Design review of the part built by this model. Coordinates are the model's own, in mm. A direction names the side the tool comes from. Coordinates: 2 decimals unless noted, no trailing zeros. Loops run counter-clockwise (first coordinate to the right, second up) from the corner with the lowest first, then second, coordinate; pieces in that order, holes last. Notation, with made-up numbers: M 83,66.5 L 124,66.5 A25 ccw 124,85.5 Z; hole C -6.75,12 d1. An arc over 180 degrees is marked long. Put each result on its own line as item: value. Start each with the question number.
(1) Take a section at C-C, the plane x = -53.5. Give the boundary of the cut face in (y, z).
(2) For faces 4 (the cylindrical face through (-48.91, -21.07, 7.19)), 5 (the flat face through (52, -28, 23.5)), 6 (the flat face through (-1, -33.4, 22)), list the 3-axis set-ups (+Z, -Z, +X, -X, +Y, -Y) from which the entire face can be reached by the end or side of a thin tool; tool diameter is ignored.
(3) For probe 1 along X at (y, z) = (-22, 6); probe 2 along X at (y, z) = (0, 2.05); probe 3 along Y at (x, z) = (51.5, 22), list the stretches that pass through material, from the lowest coordinate up. Write a range as [from, to].
(4) The part is to be moulded in two halves that separate along X. For faces 1 (the cylindrical face through (-43.624, 22.024, 7.19)), 2 (the cylindrical face through (57.321, 0.22, 27.745)), 3 (the flat face through (-49.34, 23.03, 11.5)), say which applies: +X half, -X half, draft (parallel to the pull), parting line (faces both ways), or undercut.
(5) Clearance check with flat-ended pins moving along their axes: pin 1 (2.5 mm diameter, centred on x = -49.5, y = -22.5, fed in from +Z); pin 2 (6 mm diameter, centred on x = 20, y = 20, fed in from +Z); pin 3 (3 mm diameter, centred on x = 53.5, y = 28.1, fed in from +Z); pin 4 (2 mm diameter, centred on x = -48.8, y = 0, fed in from -Z). State where each tip first meets the part, or that it passes through.
(6) Take a section at A-A, the plane z = 9. Count the separate pieces of the cut face and the enclosed holes in it, then the cut area to 3 significant figures.
(7) Take a section at D-D, the plane y = 28.1. Give the boundary of the cut face in (x, z).
(8) Take a section at B-B, the plane z = 36.5. Give the boundary of the cut face in (x, y).
```python
from build123d import *

# Parameters (mm, degrees)
SCHIZZO1_W                           = 117.6
SCHIZZO1_H                           = 66.8
ESTRUSIONE_ESTRUSIONE1_DEPTH         = 3
SCHIZZO2_W                           = 117.6
SCHIZZO2_H                           = 66.8
SCHIZZO2_W_2                         = 111.6
SCHIZZO2_H_2                         = 60.8
ESTRUSIONE_FORI_COVER_DEPTH          = 40.5
SCHIZZO4_R                           = 4
SCHIZZO4_R_2                         = 1.75
ESTRUSIONE_FORI_PCB_DEPTH            = 8.5
SCHIZZO7_R                           = 3.5
ESTRUSIONE_FORI_CHASSIS_DEPTH        = 1
SCHIZZO8_R                           = 1.85
TAGLIO_ESTRUSIONE2_DEPTH             = 79.82417142
TAGLIO_ESTRUSIONE2_DIRECTION_2_REACH = 80.824
RACCORDO3_R                          = 2
RACCORDO4_R                          = 2
RACCORDO5_R                          = 2
RACCORDO6_R                          = 2
RACCORDO7_R                          = 2
SCHIZZO9_R                           = 1.2
ESTRUSIONE_ESTRUSIONE6_DEPTH         = 20
TAGLIO_FORO_CAVI_REACH               = 131.76
SCHIZZO11_R                          = 5


with BuildPart() as part:
    # Schizzo1 → Estrusione-Estrusione1 (new body)
    with BuildSketch(Plane.XY):
        Rectangle(SCHIZZO1_W, SCHIZZO1_H)
    extrude(amount=ESTRUSIONE_ESTRUSIONE1_DEPTH)

    # Schizzo2 → Estrusione- Fori Cover (add)
    with BuildSketch(Plane.XY.offset(3)):
        Rectangle(SCHIZZO2_W, SCHIZZO2_H)
        Rectangle(SCHIZZO2_W_2, SCHIZZO2_H_2, mode=Mode.SUBTRACT)
    extrude(amount=ESTRUSIONE_FORI_COVER_DEPTH)

    # Schizzo4 → Estrusione- Fori PCB (add)
    # profile 1 of 4: a face of its own
    with BuildSketch(Plane.XY.offset(3)):
        with Locations(Location((-47.62, 22.2, 0), (0, 0, 180))):
            Circle(SCHIZZO4_R)
        with Locations((-47.62, 22.2)):
            Circle(SCHIZZO4_R_2, mode=Mode.SUBTRACT)
    # profile 2 of 4: a face of its own
    with BuildSketch(Plane.XY.offset(3)):
        with Locations(Location((47.63, 22.2, 0), (0, 0, 180))):
            Circle(SCHIZZO4_R)
        with Locations((47.63, 22.2)):
            Circle(SCHIZZO4_R_2, mode=Mode.SUBTRACT)
    # profile 3 of 4: a face of its own
    with BuildSketch(Plane.XY.offset(3)):
        with Locations(Location((47.63, -22.25, 0), (0, 0, 180))):
            Circle(SCHIZZO4_R)
        with Locations((47.63, -22.25)):
            Circle(SCHIZZO4_R_2, mode=Mode.SUBTRACT)
    # profile 4 of 4: a face of its own
    with BuildSketch(Plane.XY.offset(3)):
        with Locations(Location((-47.62, -22.25, 0), (0, 0, 180))):
            Circle(SCHIZZO4_R)
        with Locations((-47.62, -22.25)):
            Circle(SCHIZZO4_R_2, mode=Mode.SUBTRACT)
    extrude(amount=ESTRUSIONE_FORI_PCB_DEPTH)

    # Schizzo7 → Estrusione-Fori Chassis (add)
    with BuildSketch(Plane.XY.offset(3)):
        with Locations(Location((-48.8, 0, 0), (0, 0, 180))):
            Circle(SCHIZZO7_R)
        with Locations(Location((48.8, 0, 0), (0, 0, 180))):
            Circle(SCHIZZO7_R)
    extrude(amount=ESTRUSIONE_FORI_CHASSIS_DEPTH)

    # Schizzo8 → Taglio-Estrusione2 (cut)
    with BuildSketch(Plane.XY.offset(3)):
        with Locations((-48.8, 0)):
            Circle(SCHIZZO8_R)
        with Locations((48.8, 0)):
            Circle(SCHIZZO8_R)
    extrude(amount=-TAGLIO_ESTRUSIONE2_DEPTH, mode=Mode.SUBTRACT)

    # Schizzo8 → Taglio-Estrusione2 direction 2 (cut, up to next)
    with BuildSketch(Plane.XY.offset(3), mode=Mode.PRIVATE) as taglio_estrusione2_direction_2_sk1:
        with Locations((-48.8, 0)):
            Circle(SCHIZZO8_R)
    taglio_estrusione2_direction_2_tool1 = extrude(taglio_estrusione2_direction_2_sk1.sketch, amount=TAGLIO_ESTRUSIONE2_DIRECTION_2_REACH, mode=Mode.PRIVATE) & part.part
    # Schizzo8 → Taglio-Estrusione2 direction 2 (cut, up to next)
    with BuildSketch(Plane.XY.offset(3), mode=Mode.PRIVATE) as taglio_estrusione2_direction_2_sk2:
        with Locations((48.8, 0)):
            Circle(SCHIZZO8_R)
    taglio_estrusione2_direction_2_tool2 = extrude(taglio_estrusione2_direction_2_sk2.sketch, amount=TAGLIO_ESTRUSIONE2_DIRECTION_2_REACH, mode=Mode.PRIVATE) & part.part
    add(taglio_estrusione2_direction_2_tool1.solids().sort_by_distance((-48.8, 0, 3))[0], mode=Mode.SUBTRACT)
    add(taglio_estrusione2_direction_2_tool2.solids().sort_by_distance((48.8, 0, 3))[0], mode=Mode.SUBTRACT)

    # Raccordo3
    raccordo3_edges = [part.edges().sort_by_distance(p)[0] for p in [
        (-58.8, 33.4, 21.75),
    ]]
    fillet(raccordo3_edges, radius=RACCORDO3_R)

    # Raccordo4
    raccordo4_edges = [part.edges().sort_by_distance(p)[0] for p in [
        (58.8, 33.4, 21.75),
    ]]
    fillet(raccordo4_edges, radius=RACCORDO4_R)

    # Raccordo5
    raccordo5_edges = [part.edges().sort_by_distance(p)[0] for p in [
        (-58.8, -33.4, 21.75),
    ]]
    fillet(raccordo5_edges, radius=RACCORDO5_R)

    # Raccordo6
    raccordo6_edges = [part.edges().sort_by_distance(p)[0] for p in [
        (58.8, -33.4, 21.75),
    ]]
    fillet(raccordo6_edges, radius=RACCORDO6_R)

    # Raccordo7
    raccordo7_edges = [part.edges().sort_by_distance(p)[0] for p in [
        (0, -33.4, 0),
        (-58.214213562, -32.814213562, 0),
        (58.8, 0, 0),
        (58.214213562, -32.814213562, 0),
        (-58.8, 0, 0),
        (-58.214213562, 32.814213562, 0),
        (0, 33.4, 0),
        (58.214213562, 32.814213562, 0),
    ]]
    fillet(raccordo7_edges, radius=RACCORDO7_R)

    # Schizzo9 → Estrusione-Estrusione6 (add)
    # profile 1 of 4: a face of its own
    with BuildSketch(Plane.XY.offset(43.5)):
        with BuildLine():
            Line((-55.8, 24.4), (-55.8, 30.4))
            Line((-55.8, 30.4), (-49.8, 30.4))
            ThreePointArc((-49.8, 30.4), (-51.557359313, 26.157359313), (-55.8, 24.4))
        make_face()
        with Locations((-53.5, 28.1)):
            Circle(SCHIZZO9_R, mode=Mode.SUBTRACT)
    # profile 2 of 4: a face of its own
    with BuildSketch(Plane.XY.offset(43.5)):
        with BuildLine():
            Line((49.8, 30.4), (55.8, 30.4))
            Line((55.8, 30.4), (55.8, 24.4))
            ThreePointArc((55.8, 24.4), (51.557359313, 26.157359313), (49.8, 30.4))
        make_face()
        with Locations((53.5, 28.1)):
            Circle(SCHIZZO9_R, mode=Mode.SUBTRACT)
    # profile 3 of 4: a face of its own
    with BuildSketch(Plane.XY.offset(43.5)):
        with BuildLine():
            Line((55.8, -24.4), (55.8, -30.4))
            Line((55.8, -30.4), (49.8, -30.4))
            ThreePointArc((49.8, -30.4), (51.557359313, -26.157359313), (55.8, -24.4))
        make_face()
        with Locations((53.5, -28.1)):
            Circle(SCHIZZO9_R, mode=Mode.SUBTRACT)
    # profile 4 of 4: a face of its own
    with BuildSketch(Plane.XY.offset(43.5)):
        with BuildLine():
            Line((-55.8, -24.4), (-55.8, -30.4))
            Line((-55.8, -30.4), (-49.8, -30.4))
            ThreePointArc((-49.8, -30.4), (-51.557359313, -26.157359313), (-55.8, -24.4))
        make_face()
        with Locations((-53.5, -28.1)):
            Circle(SCHIZZO9_R, mode=Mode.SUBTRACT)
    extrude(amount=-ESTRUSIONE_ESTRUSIONE6_DEPTH)

    # Schizzo11 → Taglio- Foro Cavi (cut, up to next)
    with BuildSketch(Plane(origin=(58.8, 0, 0), x_dir=(0, 0, -1), z_dir=(1, 0, 0)), mode=Mode.PRIVATE) as taglio_foro_cavi_sk1:
        with Locations((-22.75, 0)):
            Circle(SCHIZZO11_R)
    taglio_foro_cavi_tool1 = extrude(taglio_foro_cavi_sk1.sketch, amount=-TAGLIO_FORO_CAVI_REACH, mode=Mode.PRIVATE) & part.part
    add(taglio_foro_cavi_tool1.solids().sort_by_distance((58.8, 0, 22.75))[0], mode=Mode.SUBTRACT)


solid = part.part
```
Computed values:
1. outline: M -33.4,2 A2 ccw -31.4,0 L 31.4,0 A2 ccw 33.4,2 L 33.4,43.5 L 29.3,43.5 L 29.3,23.5 L 30.4,23.5 L 30.4,3 L -30.4,3 L -30.4,23.5 L -29.3,23.5 L -29.3,43.5 L -33.4,43.5 Z; M -26.9,23.5 L -24.86,23.5 L -24.86,43.5 L -26.9,43.5 Z; M 24.86,23.5 L 26.9,23.5 L 26.9,43.5 L 24.86,43.5 Z
2. face 4: +Z
2. face 5: none
2. face 6: +Z, -Z, +X, -X, -Y
3. probe 1: x = [-58.8, -55.8], [-51.61, -49.35], [-45.89, -43.63], [43.64, 45.9], [49.36, 51.62], [55.8, 58.8]
3. probe 2: x = [-58.8, -50.65], [-46.95, 46.95], [50.65, 58.8]
3. probe 3: y = [-33.4, -30.4], [30.4, 33.4]
4. face 1: undercut
4. face 2: draft
4. face 3: undercut
5. pin 1: stops at z = 11.5
5. pin 2: stops at z = 3
5. pin 3: stops at z = 43.5
5. pin 4: passes through
6. separate pieces: 5
6. enclosed holes: 5
6. area: 1,230 mm^2
7. outline: M -58.8,2 A2 ccw -56.8,0 L 56.8,0 A2 ccw 58.8,2 L 58.8,43.5 L 54.7,43.5 L 54.7,23.5 L 55.8,23.5 L 55.8,3 L -55.8,3 L -55.8,23.5 L -54.7,23.5 L -54.7,43.5 L -58.8,43.5 Z; M -52.3,23.5 L -50.26,23.5 L -50.26,43.5 L -52.3,43.5 Z; M 50.26,23.5 L 52.3,23.5 L 52.3,43.5 L 50.26,43.5 Z
8. outline: M -58.8,-31.4 A2 ccw -56.8,-33.4 L 56.8,-33.4 A2 ccw 58.8,-31.4 L 58.8,31.4 A2 ccw 56.8,33.4 L -56.8,33.4 A2 ccw -58.8,31.4 Z; hole M -55.8,-24.4 A6 cw -49.8,-30.4 L 49.8,-30.4 A6 cw 55.8,-24.4 L 55.8,24.4 A6 cw 49.8,30.4 L -49.8,30.4 A6 cw -55.8,24.4 Z; hole C -53.5,-28.1 d2.4; hole C -53.5,28.1 d2.4; hole C 53.5,-28.1 d2.4; hole C 53.5,28.1 d2.4
